Can you work these out from the model? Positions are in its coordinate system, mm. Face numbers are marked on the shaded views. Give positions to 0.01 mm unless a question says otherwise; leave off trailing zeros. Loops run counter-clockwise (first coordinate to the right, second up) from the corner with the lowest first, then second, coordinate; pieces in that order, holes last. Notation, with made-up numbers: (-4.75, 28) - (50.25, 28) arc R8 ccw to (50.25, 42) - close; hole circle Ø4 at (-31, -37.75). An arc over 180 degrees is marked (long way). Answer as a JSON object with one key per item and string values. Group by question number.
Item 1: Suppose I cut it at C-C on y = 10. Write out the boundary of the cut face in (x, z).
Item 2: Suppose I cut it at D-D on x = -28. Write out the boundary of the cut face in (y, z).
Item 3: Will these pins go through, and if not, where does the flat tip stop? pin 1 (10 mm diameter, centred on x = -19, z = -53.5, fed in from +Y); pin 2 (1.2 mm diameter, centred on x = -44, y = 3, fed in from -Z); pin 3 (1.2 mm diameter, centred on x = -32.5, y = 1.5, fed in from +Z).
Item 4: Suppose I cut it at B-B on y = 2. Write out the boundary of the cut face in (x, z).
Item 5: Thinking about a two-plate mould opening in X: for the marked faces 1 and 2, which applies, pulls with the +X half, pulls with the -X half, needs draft (parallel to the pull), parting line crosses it, or undercut?
Item 6: Suppose I cut it at A-A on z = -66. Write out the boundary of the cut face in (x, y).
Item 7: Please list where these lines run through material, in increasing order: L1, parallel to X at y = 1.5, z = -100; L2, parallel to Y at x = -28, z = -86; L3, parallel to Z at x = -67.5, y = 3.
from build123d import *

# Parameters (mm, degrees)
SKETCH3_W           = 12
SKETCH3_H           = 80
SKETCH3_W_2         = 50
SKETCH3_H_2         = 10.001862112
BOSS_EXTRUDE1_DEPTH = 4
SKETCH4_R           = 3.5
SKETCH4_R_2         = 2
BOSS_EXTRUDE2_DEPTH = 7


with BuildPart() as part:
    # Sketch3 → Boss-Extrude1 (new body)
    with BuildSketch(Plane(origin=(0, 0, 0), x_dir=(1, 0, 0), z_dir=(0, 1, 0))):
        with Locations((-75.710799504, 83.763400912)):
            Rectangle(SKETCH3_W, SKETCH3_H)
        with Locations((-44.710799504, 83.763400912)):
            Rectangle(SKETCH3_W_2, SKETCH3_H_2)
        with Locations((-13.710799504, 83.763400912)):
            Rectangle(SKETCH3_W, SKETCH3_H)
    extrude(amount=BOSS_EXTRUDE1_DEPTH)

    # Sketch4 → Boss-Extrude2 (add)
    # profile 1 of 2: a face of its own
    with BuildSketch(Plane(origin=(0, 4, 0), x_dir=(1, 0, 0), z_dir=(0, 1, 0))):
        with Locations(Location((-75.710799504, 83.763400912, 0), (0, 0, 270))):
            Circle(SKETCH4_R)
        with Locations(Location((-75.710799504, 83.763400912, 0), (0, 0, 270))):
            Circle(SKETCH4_R_2, mode=Mode.SUBTRACT)
    # profile 2 of 2: a face of its own
    with BuildSketch(Plane(origin=(0, 4, 0), x_dir=(1, 0, 0), z_dir=(0, 1, 0))):
        with Locations(Location((-13.710799504, 83.763400912, 0), (0, 0, 270))):
            Circle(SKETCH4_R)
        with Locations(Location((-13.710799504, 83.763400912, 0), (0, 0, 270))):
            Circle(SKETCH4_R_2, mode=Mode.SUBTRACT)
    extrude(amount=BOSS_EXTRUDE2_DEPTH)


solid = part.part
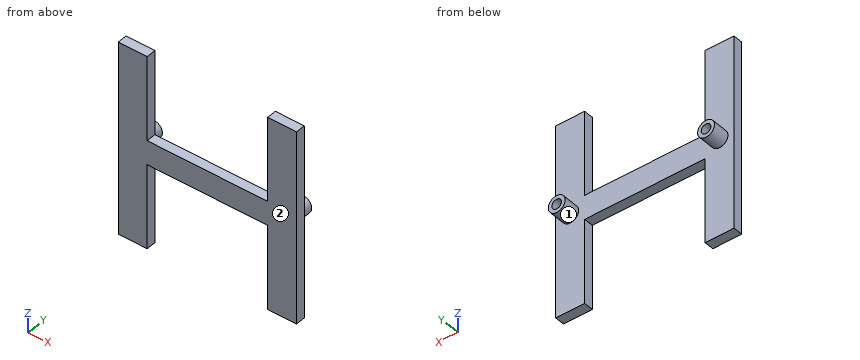
Worked out:
{
 "1": {"outline": "circle Ø7 at (-75.71, -83.76); circle Ø7 at (-13.71, -83.76); hole circle Ø4 at (-75.71, -83.76); hole circle Ø4 at (-13.71, -83.76)"},
 "2": {"outline": "(0, -88.76) - (4, -88.76) - (4, -78.76) - (0, -78.76) - close"},
 "3": {"pin 1": "stops at y = 4", "pin 2": "stops at z = -88.76", "pin 3": "stops at z = -78.76"},
 "4": {"outline": "(-81.71, -123.76) - (-69.71, -123.76) - (-69.71, -88.76) - (-19.71, -88.76) - (-19.71, -123.76) - (-7.71, -123.76) - (-7.71, -43.76) - (-19.71, -43.76) - (-19.71, -78.76) - (-69.71, -78.76) - (-69.71, -43.76) - (-81.71, -43.76) - close"},
 "5": {"face 1": "undercut", "face 2": "needs draft"},
 "6": {"outline": "(-81.71, 0) - (-69.71, 0) - (-69.71, 4) - (-81.71, 4) - close; (-19.71, 0) - (-7.71, 0) - (-7.71, 4) - (-19.71, 4) - close"},
 "7": {"L1": "x = -81.71 to -69.71, -19.71 to -7.71", "L2": "y = 0 to 4", "L3": "z = -88.76 to -78.76"}
}
